```python
from build123d import *

# Parameters (mm, degrees)
SKETCH_1_W          = 101.6
SKETCH_1_H          = 53.34
EXTRUDE_1_DEPTH     = 1.5
SKETCH_2_W          = 16
SKETCH_2_H          = 12
EXTRUDE_2_DEPTH     = 10
SKETCH_3_W          = 6
SKETCH_3_H          = 2.163495019
CUT_EXTRUDE_1_DEPTH = 10
SKETCH_6_R          = 1.75
CUT_EXTRUDE_2_DEPTH = 74.684282714


with BuildPart() as part:
    # 草图1 → 凸台-拉伸1 (new body)
    with BuildSketch(Plane(origin=(0, 0, 0), x_dir=(1, 0, 0), z_dir=(0, 1, 0))):
        with Locations((14.806341463, 5.348455285)):
            Rectangle(SKETCH_1_W, SKETCH_1_H)
    extrude(amount=EXTRUDE_1_DEPTH)

    # 草图2 → 凸台-拉伸2 (add)
    with BuildSketch(Plane(origin=(0, 1.5, 0), x_dir=(1, 0, 0), z_dir=(0, 1, 0))):
        with Locations((-36.993658537, 18.018455285)):
            Rectangle(SKETCH_2_W, SKETCH_2_H)
    extrude(amount=EXTRUDE_2_DEPTH)

    # 草图3 → 切除-拉伸1 (cut)
    with BuildSketch(Plane.ZY.offset(44.993658537)):
        Polygon((-21.018455285, 10.5), (-23.018455285, 8.5), (-23.018455285, 2.5), (-13.018455285, 2.5), (-13.018455285, 8.5), (-15.018455285, 10.5), align=None)
        with Locations((-18.018455285, 6.471327075)):
            Rectangle(SKETCH_3_W, SKETCH_3_H, mode=Mode.SUBTRACT)
    extrude(amount=-CUT_EXTRUDE_1_DEPTH, mode=Mode.SUBTRACT)

    # 草图6 → 切除-拉伸2 (cut, through all)
    with BuildSketch(Plane(origin=(0, 1.5, 0), x_dir=(1, 0, 0), z_dir=(0, 1, 0))):
        with Locations(Location((-20.753658537, 29.478455285, 0), (0, 0, 270))):
            Circle(SKETCH_6_R)
        with Locations(Location((54.176341463, 29.478455285, 0), (0, 0, 270))):
            Circle(SKETCH_6_R)
        with Locations(Location((-22.023658537, -18.781544715, 0), (0, 0, 270))):
            Circle(SKETCH_6_R)
        with Locations(Location((30.046341463, -13.701544715, 0), (0, 0, 270))):
            Circle(SKETCH_6_R)
        with Locations(Location((60.526341463, -18.781544715, 0), (0, 0, 270))):
            Circle(SKETCH_6_R)
    extrude(amount=-CUT_EXTRUDE_2_DEPTH, mode=Mode.SUBTRACT)


solid = part.part
```
The model under review builds one solid part; all positions refer to its coordinate system, in mm. A direction names the side the tool comes from. Give positions to 0.01 mm unless a question says otherwise; leave off trailing zeros. Loops run counter-clockwise (first coordinate to the right, second up) from the corner with the lowest first, then second, coordinate; pieces in that order, holes last. Notation, with made-up numbers: (40.5, 25) - (75.5, 25) arc R32 cw to (75.5, 60) - close; hole circle Ø5 at (14, 73.5). An arc over 180 degrees is marked (long way). Answer as a JSON object with one key per item and string values.
Q1. Insertion check: pin 1 (3 mm diameter, centred on x = 46.5, z = 8.5, fed in from -Y); pin 2 (5 mm diameter, centred on x = -40.5, y = 6.5, fed in from +Z); pin 3 (3 mm diameter, centred on x = -22.5, y = 3.5, fed in from -Z); pin 4 (1.1 mm diameter, centred on x = -38.5, y = 6.5, fed in from -Z). Each pin has a flat end and moves straight along its axis. Give the tip position at first contact, or say it passes through.
Worked out:
{"pin 1": "stops at y = 0", "pin 2": "stops at z = -12.02", "pin 3": "passes through", "pin 4": "stops at z = -24.02"}
Q2. For faces 1 (the flat face through (-44.994, 6, -18)), 2 (the flat face through (-40, 7.553, -18)), 3 (the flat face through (-41, 1.5, -18)), list the 3-axis set-ups (+Z, -Z, +X, -X, +Y, -Y) from which the entire face can be reached by the end or side of a thin tool; tool diameter is ignored.
Worked out:
{"face 1": "+Z, -Z, -X, +Y, -Y", "face 2": "-X", "face 3": "+Z, -Z, -X, -Y"}
Q3. Add section A-A on x = -33. State the section outline as (y, z) points, plus the area to 3 significant figures.
Worked out:
{"outline": "(0, -32.02) - (1.5, -32.02) - (1.5, -24.02) - (11.5, -24.02) - (11.5, -12.02) - (1.5, -12.02) - (1.5, 21.32) - (0, 21.32) - close", "area": "200 mm^2"}
Q4. Add section C-C on y = 4.25. State the section outline as (x, z) points, plus the area to 3 significant figures.
Worked out:
{"outline": "(-44.99, -24.02) - (-28.99, -24.02) - (-28.99, -12.02) - (-44.99, -12.02) - (-44.99, -13.02) - (-34.99, -13.02) - (-34.99, -23.02) - (-44.99, -23.02) - close", "area": "92.0 mm^2"}
Q5. Add section B-B on z = -19.5. State the section outline as (x, y) points.
Worked out:
{"outline": "(-44.99, 1.5) - (-35.99, 1.5) - (-35.99, 0) - (65.61, 0) - (65.61, 1.5) - (-28.99, 1.5) - (-28.99, 11.5) - (-44.99, 11.5) - (-44.99, 10.5) - (-34.99, 10.5) - (-34.99, 7.55) - (-44.99, 7.55) - (-44.99, 5.39) - (-34.99, 5.39) - (-34.99, 2.5) - (-44.99, 2.5) - close"}
Q6. To check wall thickness, follow line 1 along Y through (x, z) = (28, -7); line 2 along X through (y, z) = (6.25, -17); line 3 along X through (y, z) = (4.5, -13.5). State the ranges of each line that lie inside material, in increasing order.
Worked out:
{"line 1": "y = 0 to 1.5", "line 2": "x = -44.99 to -28.99", "line 3": "x = -34.99 to -28.99"}
Q7. Add section D-D on z = 13. State the section outline as (x, y) points.
Worked out:
{"outline": "(-35.99, 0) - (28.44, 0) - (28.44, 1.5) - (-35.99, 1.5) - close; (31.65, 0) - (65.61, 0) - (65.61, 1.5) - (31.65, 1.5) - close"}
Q8. Mouldability with a two-part tool opening along X and no side actions: class faces 4 (the cylindrical face through (-21.42, 0.76, -27.86)), 5 (the flat face through (-37, 6, -24.018)), 6 (the cylindrical face through (-20.29, 0.76, 18.55)), 7 (the flat face through (-28.994, 6, -18)) as +X half, -X half, draft (parallel to the pull), parting line (faces both ways), or undercut.
Worked out:
{"face 4": "undercut", "face 5": "draft", "face 6": "undercut", "face 7": "+X half"}
